Build history of the part. All positions in model axes, mm. Give positions to 0.01 mm unless a question says otherwise; leave off trailing zeros. Order: outer loops, then holes, each group sorted by start corner. A loop starts at its lowest first (then second) coordinate and runs counter-clockwise, first axis right, second up. Notation, with made-up numbers: M 18.5,-16.5 L 64.5,-16.5 A16 ccw 64.5,-8.5 Z; hole C 41.25,-38 d4. An arc over 180 degrees is marked long. One line per item, written item: value.
from build123d import *

# Parameters (mm, degrees)
SKETCH1_R               = 22.225
BOSS_EXTRUDE1_DEPTH     = 41.275
CUT_EXTRUDE1_DEPTH      = 79.673399253
CUT_EXTRUDE1_DEPTH_BACK = 79.673399253
SKETCH2_R               = 3.2639
CUT_EXTRUDE2_DEPTH      = 79.673399422
CUT_EXTRUDE2_DEPTH_BACK = 79.673399422
SKETCH3_R               = 3.2639


with BuildPart() as part:
    # Sketch1 → Boss-Extrude1 (new body)
    with BuildSketch(Plane(origin=(0, 0, 0), x_dir=(0, 1, 0), z_dir=(0, 0, 1))):
        with BuildLine():
            Line((-34.925, 0), (-34.925, -57.15))
            Line((-34.925, -57.15), (34.925, -57.15))
            Line((34.925, -57.15), (34.925, 0))
            ThreePointArc((34.925, 0), (0, 34.925), (-34.925, 0))
        make_face()
        with Locations(Location((0, 0, 0), (0, 0, 270))):
            Circle(SKETCH1_R, mode=Mode.SUBTRACT)
    extrude(amount=BOSS_EXTRUDE1_DEPTH)

    # Sketch2 → Cut-Extrude1 (cut, two sides: drawn at the far end of the back side and taken through both)
    with BuildSketch(Plane.YZ.offset(-CUT_EXTRUDE1_DEPTH_BACK)):
        with Locations(Location((0, 27.516666667, 0), (0, 0, 270))):
            Circle(SKETCH2_R)
    extrude(amount=CUT_EXTRUDE1_DEPTH + CUT_EXTRUDE1_DEPTH_BACK, mode=Mode.SUBTRACT)

    # Sketch3 → Cut-Extrude2 (cut, two sides: drawn at the far end of the back side and taken through both)
    with BuildSketch(Plane(origin=(0, 0, 0), x_dir=(-1, 0, 0), z_dir=(0, 1, 0)).offset(-CUT_EXTRUDE2_DEPTH_BACK)):
        with Locations(Location((0, 13.758333333, 0), (0, 0, 90))):
            Circle(SKETCH3_R)
    extrude(amount=CUT_EXTRUDE2_DEPTH + CUT_EXTRUDE2_DEPTH_BACK, mode=Mode.SUBTRACT)


solid = part.part
1) Saw through at C-C, the plane z = 8. Write the cut outline in (x, y) (3 decimals).
Check values:
outline: M 0,-34.925 L 57.15,-34.925 L 57.15,34.925 L 0,34.925 A34.925 ccw Z; hole C 0,0 d44.45
2) Mould opens along Z. For faces 1 (the face through (-1.25, 28.361, 16.773)), 2 (the face through (-1.25, -28.542, 16.773)), 3 (the face through (28, -34.925, 20)), 4 (the face through (21, -8, 41.275)) say: released by +Z, released by -Z, zero draft, split by the parting line, or undercut.
Check values:
face 1: undercut
face 2: undercut
face 3: zero draft
face 4: released by +Z
3) Saw through at A-A, the plane y = 0. Write the cut outline in (x, z) (3 decimals).
Check values:
outline: M -34.925,0 L -22.225,0 L -22.225,24.253 L -34.925,24.253 Z; M -34.925,30.781 L -22.225,30.781 L -22.225,41.275 L -34.925,41.275 Z; M 22.225,0 L 57.15,0 L 57.15,24.253 L 22.225,24.253 Z; M 22.225,30.781 L 57.15,30.781 L 57.15,41.275 L 22.225,41.275 Z
4) Drill centre lines: probe 1 along Z at (x, y) = (42.5, 0) (3 decimals); probe 2 along Y at (x, z) = (18, 26.5) (3 decimals); probe 3 along X at (y, z) = (7, 38). Where is each one in solid material? Low to high. Write a range as from..to.
Check values:
probe 1: 0..24.253, 30.781..41.275
probe 2: -34.925..-13.037, 13.037..34.925
probe 3: -34.22..-21.09, 21.09..57.15
5) Saw through at B-B, the plane x = -1. Write the cut outline in (y, z) (1 decimal), then the cut area to 3 significant figures.
Check values:
outline: M -34.9,0 L -22.2,0 L -22.2,10.7 L -34.9,10.7 Z; M -34.9,16.9 L -22.2,16.9 L -22.2,41.3 L -34.9,41.3 Z; M 22.2,0 L 34.9,0 L 34.9,10.7 L 22.2,10.7 Z; M 22.2,16.9 L 34.9,16.9 L 34.9,41.3 L 22.2,41.3 Z
area: 891 mm^2
6) Saw through at D-D, the plane x = -12. Write the cut outline in (y, z) (3 decimals), then the cut area to 3 significant figures.
Check values:
outline: M -32.799,0 L -18.707,0 L -18.707,41.275 L -32.799,41.275 Z; M 18.707,0 L 32.799,0 L 32.799,41.275 L 18.707,41.275 Z
area: 1,160 mm^2
7) Pin check, flat tips, straight feed: pin 1 (6 mm diameter, centred on x = 35.5, y = -15.5, fed in from -Z); pin 2 (1.5 mm diameter, centred on y = -8.5, z = 8, fed in from -X); pin 3 (5 mm diameter, centred on x = 0, z = 13.76, fed in from +Y); pin 4 (1 mm diameter, centred on x = -13, z = 32.5, fed in from -Y). Stop position of each tip, or through.
Check values:
pin 1: z = 0
pin 2: x = -34.05
pin 3: through
pin 4: y = -32.61
